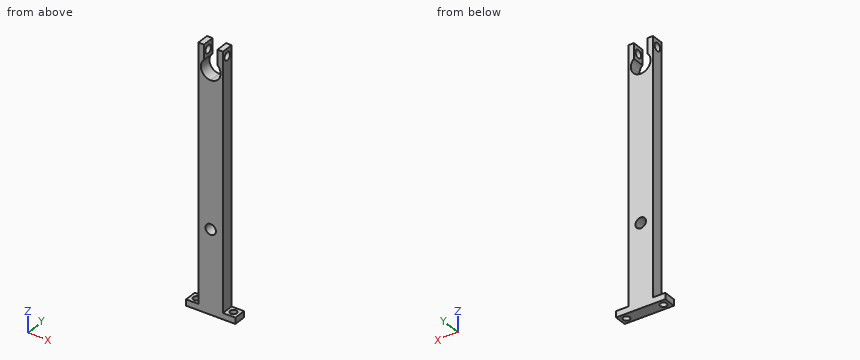
```python
from build123d import *

# Parameters (mm, degrees)
F1_DEPTH = 5
F3_DEPTH = 25
F5_DEPTH = 5


with BuildPart() as f1:
    # F0 (on Front) → F1 (new body, symmetric)
    with BuildSketch(Plane.XZ):
        with BuildLine():
            Line((-10, 105), (-10, -105))
            Line((-10, -105), (10, -105))
            Line((10, -105), (10, 105))
            Line((10, 105), (5.5, 105))
            Line((5.5, 105), (5.5, 92.809475))
            ThreePointArc((5.5, 92.809475), (7.348469, 90.162278), (8, 87))
            ThreePointArc((8, 87), (5.656854, 81.343146), (0, 79))
            ThreePointArc((0, 79), (-7.43222, 84.039916), (-5.5, 92.809475))
            Line((-5.5, 92.809475), (-5.5, 105))
            Line((-5.5, 105), (-10, 105))
        make_face()
        with BuildLine():
            ThreePointArc((4.25, -38), (-3.005204, -41.005204), (0, -33.75))
            ThreePointArc((0, -33.75), (3.005204, -34.994796), (4.25, -38))
        make_face(mode=Mode.SUBTRACT)
    extrude(amount=F1_DEPTH, both=True)

    # F2 (on face) → F3 (cut)
    with BuildSketch(Plane.YZ.offset(10)):
        with BuildLine():
            ThreePointArc((0, 102.25), (-2.298097, 96.701903), (3.25, 99))
            ThreePointArc((3.25, 99), (2.298097, 101.298097), (0, 102.25))
        make_face()
    extrude(amount=-F3_DEPTH, mode=Mode.SUBTRACT)

    # F4 (on face) → F5 (join)
    with BuildSketch(Plane(origin=(0, 0, -105), x_dir=(1, 0, 0), z_dir=(0, 0, -1))):
        with BuildLine():
            ThreePointArc((-12.25, 0), (-13.055456, 1.944544), (-15, 2.75))
            ThreePointArc((-15, 2.75), (-16.944544, -1.944544), (-12.25, 0))
        make_face()
        Polygon((-10, -5), (-10, 5), (-15, 5), (-20, 5), (-20, -5), align=None)
        with BuildLine():
            ThreePointArc((-12.25, 0), (-16.944544, -1.944544), (-15, 2.75))
            ThreePointArc((-15, 2.75), (-13.055456, 1.944544), (-12.25, 0))
        make_face(mode=Mode.SUBTRACT)
        with BuildLine():
            ThreePointArc((17.75, 0), (16.944544, 1.944544), (15, 2.75))
            ThreePointArc((15, 2.75), (13.055456, -1.944544), (17.75, 0))
        make_face()
        Polygon((15, 5), (10, 5), (10, -5), (20, -5), (20, 5), align=None)
        with BuildLine():
            ThreePointArc((17.75, 0), (13.055456, -1.944544), (15, 2.75))
            ThreePointArc((15, 2.75), (16.944544, 1.944544), (17.75, 0))
        make_face(mode=Mode.SUBTRACT)
    extrude(amount=-F5_DEPTH)


solid = f1.part
```
Source: CAD feature listing. Evaluate the final solid. Frame: model axes, mm. Give positions to 0.01 mm unless a question says otherwise; leave off trailing zeros. Loops run counter-clockwise (first coordinate to the right, second up) from the corner with the lowest first, then second, coordinate; pieces in that order, holes last. Notation, with made-up numbers: (71, 0) - (81, 0) arc R31 cw to (81, 34) - close; hole circle Ø8 at (20, 0.25). An arc over 180 degrees is marked (long way). Use CSV: the item, a comma, the result in double quotes. Start each with the question number.
1. Section B-B (z = 2.5). Output: boundary loops of the cut face in (x, y).
2. Pin query (flat end, axial travel): pin 1 (3 mm diameter, centred on x = -12, z = 74, fed in from +Y); pin 2 (5 mm diameter, centred on y = 0.5, z = -44.5, fed in from -X); pin 3 (6 mm diameter, centred on x = -12, y = -1.5, fed in from +Z); pin 4 (3 mm diameter, centred on x = -15, y = -1.5, fed in from +Z). Return the tip coordinate at first contact, or that it passes through.
3. Section A-A (z = 81.5). Output: boundary loops of the cut face in (x, y).
4. Ray query, L1, parallel to X at y = 0, z = -103.8; L2, parallel to X at y = 2, z = -38; L3, parallel to Z at x = 0, y = -0.5. Return the intervals inside material, ascending.
Response:
1,outline,"(-10, -5) - (10, -5) - (10, 5) - (-10, 5) - close"
2,pin 1,"through"
2,pin 2,"x = -10"
2,pin 3,"z = 105"
2,pin 4,"z = -100"
3,outline,"(-10, -5) - (-5.81, -5) - (-5.81, 5) - (-10, 5) - close; (5.81, -5) - (10, -5) - (10, 5) - (5.81, 5) - close"
4,L1,"-20 to -17.75, -12.25 to 12.25, 17.75 to 20"
4,L2,"-10 to -4.25, 4.25 to 10"
4,L3,"-105 to -42.25, -33.75 to 79"
